from build123d import *

# Parameters (mm, degrees)
SKETCH1_W             = 40
SKETCH1_H             = 62.5
BOSS_EXTRUDE1_DEPTH   = 15
SKETCH2_R             = 11.5
CUT_EXTRUDE1_DEPTH    = 5
SKETCH3_R             = 5.5
CUT_EXTRUDE2_DEPTH    = 71.222859526
M4_TAPPED_HOLE1_D     = 3.3
M4_TAPPED_HOLE1_DEPTH = 11.5
M4_TAPPED_HOLE1_TIP   = 0.991420021
M3_TAPPED_HOLE2_D     = 2.5
SKETCH9_W             = 40
SKETCH9_H             = 1
CUT_EXTRUDE4_DEPTH    = 73.154348448


with BuildPart() as part:
    # Sketch1 → Boss-Extrude1 (new, symmetric)
    with BuildSketch(Plane.XY):
        with Locations((0, 31.25)):
            Rectangle(SKETCH1_W, SKETCH1_H)
    extrude(amount=BOSS_EXTRUDE1_DEPTH, both=True)

    # Sketch2 → Cut-Extrude1 (cut)
    with BuildSketch(Plane.XY.offset(15)):
        with Locations((0, 13)):
            Circle(SKETCH2_R)
    extrude(amount=-CUT_EXTRUDE1_DEPTH, mode=Mode.SUBTRACT)

    # Sketch3 → Cut-Extrude2 (cut, through all)
    with BuildSketch(Plane.XY.offset(10)):
        with Locations((0, 13)):
            Circle(SKETCH3_R)
    extrude(amount=-CUT_EXTRUDE2_DEPTH, mode=Mode.SUBTRACT)

    # M4 Tapped Hole1
    with Locations(Plane(origin=(0, 62.5, 0), x_dir=(1, 0, 0), z_dir=(0, 1, 0))):
        with Locations((-15, 7.5), (15, 7.5), (15, -7.5), (-15, -7.5)):
            Hole(M4_TAPPED_HOLE1_D / 2, depth=M4_TAPPED_HOLE1_DEPTH)
            with Locations((0, 0, -(M4_TAPPED_HOLE1_DEPTH + M4_TAPPED_HOLE1_TIP / 2))):  # 118° drill point
                Cone(0, M4_TAPPED_HOLE1_D / 2, M4_TAPPED_HOLE1_TIP, mode=Mode.SUBTRACT)

    # M3 Tapped Hole2 (through all)
    with Locations(Plane.XY.offset(10)):
        with Locations((0, 13), (0, 21), (0, 5), (-8, 13), (8, 13)):
            Hole(M3_TAPPED_HOLE2_D / 2)

    # Sketch9 → Cut-Extrude4 (cut, through all)
    with BuildSketch(Plane.XY.offset(15)):
        with Locations((0, 0.5)):
            Rectangle(SKETCH9_W, SKETCH9_H)
    extrude(amount=-CUT_EXTRUDE4_DEPTH, mode=Mode.SUBTRACT)


solid = part.part
Geometry check sheet. Reference: the model listing, model coordinates, mm. A direction names the side the tool comes from. Give positions to 0.01 mm unless a question says otherwise; leave off trailing zeros. Write each loop counter-clockwise with the first axis right and the second up, starting at its lowest first coordinate (ties: lowest second). Pieces come first, ordered by that corner, then holes.
1) Cross-section at C-C (z = -4). Record the boundary of the cut face in (x, y), plus the area to 3 significant figures.
Values follow:
outline: (-20, 1) - (20, 1) - (20, 62.5) - (-20, 62.5) - close; hole circle Ø2.5 at (-8, 13); hole circle Ø11 at (0, 13); hole circle Ø2.5 at (0, 5); hole circle Ø2.5 at (0, 21); hole circle Ø2.5 at (8, 13)
area: 2,350 mm2
2) Cross-section at B-B (y = 5). Record the boundary of the cut face in (x, z), plus the area to 3 significant figures.
Values follow:
outline: (-20, -15) - (-1.25, -15) - (-1.25, 10) - (-8.26, 10) - (-8.26, 15) - (-20, 15) - close; (1.25, -15) - (20, -15) - (20, 15) - (8.26, 15) - (8.26, 10) - (1.25, 10) - close
area: 1,050 mm2
3) Thickness scan on line 1 (X direction, y = 55.75, z = 7.5); line 2 (Y direction, x = 0, z = 12.05); line 3 (Z direction, x = -15, y = 53.75). Record the ranges inside material, lowest first.
Values follow:
line 1: x = -20 to -16.65, -13.35 to 13.35, 16.65 to 20
line 2: y = 1 to 1.5, 24.5 to 62.5
line 3: z = -15 to -9.15, -5.85 to 5.85, 9.15 to 15
4) Cross-section at D-D (x = 8). Record the boundary of the cut face in (y, z), plus the area to 3 significant figures.
Values follow:
outline: (1, -15) - (11.75, -15) - (11.75, 10) - (4.74, 10) - (4.74, 15) - (1, 15) - close; (14.25, -15) - (62.5, -15) - (62.5, 15) - (21.26, 15) - (21.26, 10) - (14.25, 10) - close
area: 1,700 mm2
5) Cross-section at A-A (x = 0). Record the boundary of the cut face in (y, z), plus the area to 3 significant figures.
Values follow:
outline: (1, -15) - (3.75, -15) - (3.75, 10) - (1.5, 10) - (1.5, 15) - (1, 15) - close; (6.25, -15) - (7.5, -15) - (7.5, 10) - (6.25, 10) - close; (18.5, -15) - (19.75, -15) - (19.75, 10) - (18.5, 10) - close; (22.25, -15) - (62.5, -15) - (62.5, 15) - (24.5, 15) - (24.5, 10) - (22.25, 10) - close
area: 1,330 mm2
6) Set-up check for faces 1 (the face through (0, 39, 15)), 2 (the face through (13.476, 56.67, -6.868)): record each of +Z, -Z, +X, -X, +Y, -Y from which the full face is reachable in a straight line by a thin tool's end or side.
Values follow:
face 1: +Z, +X, -X, +Y, -Y
face 2: +Y
7) Go/stop test with flat-tipped pins: pin 1 Ø2 at (x, z) = (15, -7.5) entering from +Y; pin 2 Ø11.5 at (x, y) = (1, 18) entering from +Z. Record where each tip stops, or that it passes through.
Values follow:
pin 1: stops at y = 50.61
pin 2: stops at z = 10
8) Release check for a two-part mould opening along Z. For faces 3 (the face through (15.3, 50.2, 7.4)), 4 (the face through (-3, 8, 10)), 5 (the face through (-16.524, 56.67, 8.132)), 6 (the face through (-1.5, 24.4, 12.5)) record: released by +Z, released by -Z, zero draft, split by the parting line, or undercut.
Values follow:
face 3: undercut
face 4: released by +Z
face 5: undercut
face 6: zero draft
